Input: part model. Units: mm. Frame: model coordinates. A direction names the side the tool comes from. Coordinates: 2 decimals unless noted, no trailing zeros. Loops run counter-clockwise (first coordinate to the right, second up) from the corner with the lowest first, then second, coordinate; pieces in that order, holes last.
Item 1: Section A-A on x = 35. Return loops of the section in (y, z).
Item 2: Contact query for flat-ended pins moving along their axis: P1, Ø0.8, axis at x = -2.5, z = -0.5, coming from the -Y side; P2, Ø0.5, axis at y = 3, z = 0.5, coming from the +X side; P3, Ø1.1, axis at x = 8, z = -0.5, coming from the +Y side; P4, Ø1.9, axis at x = 35, y = -15, coming from the -Z side. Output: stop coordinate, or through.
Item 3: Ray query, line 1 along Y through (x, z) = (-35, -0.65); line 2 along Y through (x, z) = (-35, -1.55); line 3 along Y through (x, z) = (9.5, 0.65). Return the intervals inside material, ascending.
Item 4: Reachability of faces 1 (the cylindrical face through (31.147, -11.217, 0.493)), 2 (the cylindrical face through (-37.59, -17.5, -0.49)), 3 (the cylindrical face through (31.217, 11.147, 0.493)), 4 (the cylindrical face through (-31.147, 11.217, 0.493)) from +Z, -Z, +X, -X, +Y, -Y: full face, straight path, thin tool, end or side. Return the list, or none.
Item 5: Section C-C on y = -1. Return loops of the section in (x, z), and give its area (3 significant figures).
Item 6: Pull-direction query (Y, two-part tool) for faces 5 (the cylindrical face through (-31.217, -11.147, 0.493)), 6 (the cylindrical face through (35.208, -16.586, -0.986)), 7 (the flat face through (-1, 13, 0)); classes: released by +Y, released by -Y, zero draft, split by the parting line, or undercut.
Item 7: Section D-D on x = -8. Return loops of the section in (y, z), and give its area (3 significant figures).
Item 8: Section B-B on y = -15. Return loops of the section in (x, z).
```python
from build123d import *

# Parameters (mm, degrees)
SKETCH1_R           = 1.6
BOSS_EXTRUDE1_DEPTH = 2
BOSS_EXTRUDE2_DEPTH = 1
CHAMFER1_SIZE       = 1


with BuildPart() as part:
    # Sketch1 → Boss-Extrude1 (new body)
    with BuildSketch(Plane.XY):
        with BuildLine():
            Line((38, -8), (38, 8))
            ThreePointArc((38, 8), (37.945323743, 9.044287145), (37.781892872, 10.077154747))
            ThreePointArc((37.781892872, 10.077154747), (37.714830787, 11.762378479), (38.211886222, 13.374027399))
            ThreePointArc((38.211886222, 13.374027399), (37.545584412, 17.545584412), (33.374027399, 18.211886222))
            ThreePointArc((33.374027399, 18.211886222), (31.762378479, 17.714830787), (30.077154747, 17.781892872))
            ThreePointArc((30.077154747, 17.781892872), (29.044287145, 17.945323743), (28, 18))
            Line((28, 18), (-28, 18))
            ThreePointArc((-28, 18), (-29.044287145, 17.945323743), (-30.077154747, 17.781892872))
            ThreePointArc((-30.077154747, 17.781892872), (-31.762378479, 17.714830787), (-33.374027399, 18.211886222))
            ThreePointArc((-33.374027399, 18.211886222), (-37.545584412, 17.545584412), (-38.211886222, 13.374027399))
            ThreePointArc((-38.211886222, 13.374027399), (-37.714830787, 11.762378479), (-37.781892872, 10.077154747))
            ThreePointArc((-37.781892872, 10.077154747), (-37.945323743, 9.044287145), (-38, 8))
            Line((-38, 8), (-38, -8))
            ThreePointArc((-38, -8), (-37.945323743, -9.044287145), (-37.781892872, -10.077154747))
            ThreePointArc((-37.781892872, -10.077154747), (-37.714830787, -11.762378479), (-38.211886222, -13.374027399))
            ThreePointArc((-38.211886222, -13.374027399), (-37.545584412, -17.545584412), (-33.374027399, -18.211886222))
            ThreePointArc((-33.374027399, -18.211886222), (-31.762378479, -17.714830787), (-30.077154747, -17.781892872))
            ThreePointArc((-30.077154747, -17.781892872), (-29.044287145, -17.945323743), (-28, -18))
            Line((-28, -18), (28, -18))
            ThreePointArc((28, -18), (29.044287145, -17.945323743), (30.077154747, -17.781892872))
            ThreePointArc((30.077154747, -17.781892872), (31.762378479, -17.714830787), (33.374027399, -18.211886222))
            ThreePointArc((33.374027399, -18.211886222), (37.545584412, -17.545584412), (38.211886222, -13.374027399))
            ThreePointArc((38.211886222, -13.374027399), (37.714830787, -11.762378479), (37.781892872, -10.077154747))
            ThreePointArc((37.781892872, -10.077154747), (37.945323743, -9.044287145), (38, -8))
        make_face()
        with Locations((35, 15)):
            Circle(SKETCH1_R, mode=Mode.SUBTRACT)
        with Locations(Location((-35, 15, 0), (0, 0, 180))):
            Circle(SKETCH1_R, mode=Mode.SUBTRACT)
        with Locations(Location((35, -15, 0), (0, 0, 180))):
            Circle(SKETCH1_R, mode=Mode.SUBTRACT)
        with Locations((-35, -15)):
            Circle(SKETCH1_R, mode=Mode.SUBTRACT)
    extrude(amount=-BOSS_EXTRUDE1_DEPTH)

    # Sketch1_3 → Boss-Extrude2 (add)
    with BuildSketch(Plane.XY):
        with BuildLine():
            Line((-28, -12.5), (28, -12.5))
            ThreePointArc((28, -12.5), (31.181980515, -11.181980515), (32.5, -8))
            Line((32.5, -8), (32.5, 8))
            ThreePointArc((32.5, 8), (31.181980515, 11.181980515), (28, 12.5))
            Line((28, 12.5), (-28, 12.5))
            ThreePointArc((-28, 12.5), (-31.181980515, 11.181980515), (-32.5, 8))
            Line((-32.5, 8), (-32.5, -8))
            ThreePointArc((-32.5, -8), (-31.181980515, -11.181980515), (-28, -12.5))
        make_face()
    extrude(amount=BOSS_EXTRUDE2_DEPTH)

    # Chamfer1
    chamfer1_edges = [part.edges().sort_by_distance(p)[0] for p in [
        (-29.044287145, 17.945323743, -2),
        (-31.762378479, 17.714830787, -2),
        (-37.545584412, 17.545584412, -2),
        (-37.714830787, 11.762378479, -2),
        (-37.945323743, 9.044287145, -2),
        (-38, 0, -2),
        (-37.945323743, -9.044287145, -2),
        (-37.714830787, -11.762378479, -2),
        (-37.545584412, -17.545584412, -2),
        (-31.762378479, -17.714830787, -2),
        (29.044287145, 17.945323743, -2),
        (-29.044287145, -17.945323743, -2),
        (0, -18, -2),
        (29.044287145, -17.945323743, -2),
        (31.762378479, -17.714830787, -2),
        (37.545584412, -17.545584412, -2),
        (37.714830787, -11.762378479, -2),
        (37.945323743, -9.044287145, -2),
        (38, 0, -2),
        (37.945323743, 9.044287145, -2),
        (37.714830787, 11.762378479, -2),
        (0, 18, -2),
        (37.545584412, 17.545584412, -2),
        (31.762378479, 17.714830787, -2),
    ]]
    chamfer(chamfer1_edges, length=CHAMFER1_SIZE)


solid = part.part
```
Results found:
1. outline: (-18.6, -1) - (-17.6, -2) - (-16.6, -2) - (-16.6, 0) - (-18.6, 0) - close; (-13.4, -2) - (13.4, -2) - (13.4, 0) - (-13.4, 0) - close; (16.6, -2) - (17.6, -2) - (18.6, -1) - (18.6, 0) - (16.6, 0) - close
2. P1: stops at y = -18
2. P2: stops at x = 32.5
2. P3: stops at y = 18
2. P4: passes through
3. line 1: y = -18.6 to -16.6, -13.4 to 13.4, 16.6 to 18.6
3. line 2: y = -18.05 to -16.6, -13.4 to 13.4, 16.6 to 18.05
3. line 3: y = -12.5 to 12.5
4. face 1: +Z, +X, -Y
4. face 2: +Z, -Z
4. face 3: +Z, +X, +Y
4. face 4: +Z, -X, +Y
5. outline: (-38, -1) - (-37, -2) - (37, -2) - (38, -1) - (38, 0) - (32.5, 0) - (32.5, 1) - (-32.5, 1) - (-32.5, 0) - (-38, 0) - close
5. area: 216 mm2
6. face 5: released by -Y
6. face 6: undercut
6. face 7: zero draft
7. outline: (-18, -1) - (-17, -2) - (17, -2) - (18, -1) - (18, 0) - (12.5, 0) - (12.5, 1) - (-12.5, 1) - (-12.5, 0) - (-18, 0) - close
7. area: 96.0 mm2
8. outline: (-38.6, -1) - (-37.6, -2) - (-36.6, -2) - (-36.6, 0) - (-38.6, 0) - close; (-33.4, -2) - (33.4, -2) - (33.4, 0) - (-33.4, 0) - close; (36.6, -2) - (37.6, -2) - (38.6, -1) - (38.6, 0) - (36.6, 0) - close
